Can you work these out from the model? Positions are in its coordinate system, mm. Face numbers are marked on the shaded views. A direction names the side the tool comes from. Give positions to 0.01 mm unless a question says otherwise; leave off trailing zeros. Order: outer loops, then holes, each group sorted by start corner. A loop starts at its lowest first (then second) coordinate and runs counter-clockwise, first axis right, second up. Notation, with made-up numbers: M -1.5,52 L 28.5,52 A6 ccw 28.5,61 Z; hole C 1,-2 d4. An arc over 180 degrees is marked long. Answer as a JSON object with one key per item and string values.
Autodesk Inventor part; units mm, degrees
ref_plane "YZ Plane" through (0, 0, 0) normal (1, 0, 0) x (0, 1, 0)
ref_plane "XZ Plane" through (0, 0, 0) normal (0, 1, 0) x (-1, 0, 0)
ref_plane "XY Plane" through (0, 0, 0) normal (0, 0, 1) x (1, 0, 0)
sketch "Sketch1" plane through (0, 0, 0) normal (0, 1, 0) x (-1, 0, 0)
  line L0 (-110, 55) -> (110, 55)
  line L1 (110, 55) -> (110, -55)
  line L2 (110, -55) -> (-110, -55)
  line L3 (-110, -55) -> (-110, 55)
  line L4 (-110, 55) -> (110, -55) construction
  line L5 (110, 55) -> (-110, -55) construction
  line L6 (-150, 100) -> (150, 100)
  line L7 (150, 100) -> (150, -100)
  line L8 (150, -100) -> (-150, -100)
  line L9 (-150, -100) -> (-150, 100)
  line L10 (-150, 100) -> (150, -100) construction
  line L11 (150, 100) -> (-150, -100) construction
  arc A0 (150, -100) -> (150, 100) centre (108.3333, 0) ccw
  point P0 (0, 0)
  dimension "d0" = 220
  dimension "d1" = 110
  dimension "d2" = 300
  dimension "d3" = 200
extrude "Extrusion1" add sketch "Sketch1" along normal blind 90
extrude "Extrusion2" add sketch "Sketch1" against normal blind 50 contours A0 L7
properties part number "Sensor"
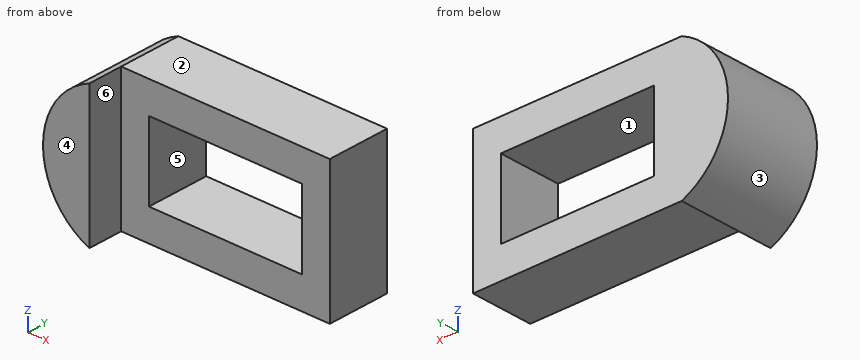
1) I need wall thicknesses on L1, parallel to Z at x = -69.5, y = 26; L2, parallel to Y at x = -126, z = 39; L3, parallel to X at y = 16, z = -16. Which ranges of each line are inside material? Lowest first, please.
Results found:
{"L1": "z = -100 to -55, 55 to 100", "L2": "y = 0 to 90", "L3": "x = -215.48 to -110, 110 to 150"}
2) I want a section at B-B on y = 36.5. Write out the boundary of the cut face in (x, z).
Results found:
{"outline": "M -150,-100 L 150,-100 L 150,100 L -150,100 A108.33 ccw Z; hole M -110,-55 L 110,-55 L 110,55 L -110,55 Z"}
3) For the marked faces 4, 5 and 6, which set-ups out of +Z, -Z, +X, -X, +Y, -Y let a thin tool reach every point of the face, with its end or its side?
Results found:
{"face 4": "+Z, -Z, +X, -X, -Y", "face 5": "+Y, -Y", "face 6": "+Z, -Z, +X, -Y"}
4) I want a section at D-D on z = 28.5. Write out the boundary of the cut face in (x, y), and give its area (3 significant figures).
Results found:
{"outline": "M -212.85,-50 L -150,-50 L -150,0 L -110,0 L -110,90 L -212.85,90 Z; M 110,0 L 150,0 L 150,90 L 110,90 Z", "area": "16,000 mm²"}
5) I want a section at A-A on x = -85. Write out the boundary of the cut face in (y, z), and give its area (3 significant figures).
Results found:
{"outline": "M 0,-100 L 90,-100 L 90,-55 L 0,-55 Z; M 0,55 L 90,55 L 90,100 L 0,100 Z", "area": "8,100 mm²"}
6) Thinking about a two-plate mould opening in X: for the marked faces 1, 2 and 3, which applies, pulls with the +X half, pulls with the -X half, needs draft (parallel to the pull), parting line crosses it, or undercut?
Results found:
{"face 1": "undercut", "face 2": "needs draft", "face 3": "pulls with the -X half"}
7) I want a section at C-C on z = -36.5. Write out the boundary of the cut face in (x, y), and give its area (3 significant figures).
Results found:
{"outline": "M -210.33,-50 L -150,-50 L -150,0 L -110,0 L -110,90 L -210.33,90 Z; M 110,0 L 150,0 L 150,90 L 110,90 Z", "area": "15,600 mm²"}
8) I'm going to push flat-ended pins straight in: pin 1 Ø15 at (y, z) = (-23, -3.5) entering from +X; pin 2 Ø4 at (y, z) = (61, 21.5) entering from -X; pin 3 Ø5 at (x, z) = (46, 55) entering from -Y. Where does each tip first touch, or does it pass through?
Results found:
{"pin 1": "stops at x = -150", "pin 2": "stops at x = -214.9", "pin 3": "stops at y = 0"}
